Read the model definition and answer for the solid it produces. Units are mm, in the model's axes. Give positions to 0.01 mm unless a question says otherwise; leave off trailing zeros. Order: outer loops, then holes, each group sorted by start corner. A loop starts at its lowest first (then second) coordinate and runs counter-clockwise, first axis right, second up. Notation, with made-up numbers: (46, -11) - (61, -11) arc R21 ccw to (61, -1) - close; hole circle Ø3 at (80, 64.5). An arc over 180 degrees is marked (long way). Write item = value, one per line.
Autodesk Inventor part; units mm, degrees
ref_plane "YZ Plane" through (0, 0, 0) normal (1, 0, 0) x (0, 1, 0)
ref_plane "XZ Plane" through (0, 0, 0) normal (0, 1, 0) x (-1, 0, 0)
ref_plane "XY Plane" through (0, 0, 0) normal (0, 0, 1) x (1, 0, 0)
sketch "Sketch1" plane through (0, 0, 0) normal (0, 1, 0) x (-1, 0, 0)
  line L0 (0, 0) -> (100, 0)
  line L1 (100, 0) -> (100, -1220)
  line L2 (100, -1220) -> (0, -1220)
  line L3 (0, -1220) -> (0, 0)
  dimension "d0" = 100
  dimension "d1" = 1220
extrude "Extrusion1" add sketch "Sketch1" along normal blind 10
ref_plane "Work Plane1" through (-50, 0, 0) normal (1, 0, 0) x (0, 0, -1)
sketch "Sketch3" plane through (-50, 0, 0) normal (1, 0, 0) x (0, 0, -1)
  line L0 (1220, 0) -> (0, 0)
  line L1 (1220, 0) -> (1220, 10)
  line L2 (0, 10) -> (1220, 10)
  line L3 (0, 0) -> (0, 10)
  line L4 (1220, 10) -> (0, 10)
  line L5 (0, 10) -> (11.15, 10)
  circle A0 centre (11.15, 120) radius 2.5
  arc A1 (15.15, 120) -> (7.15, 120) centre (11.15, 120) ccw
  line L6 (15.15, 120) -> (15.15, 10)
  line L7 (15.15, 10) -> (7.15, 10)
  line L8 (7.15, 10) -> (7.15, 120)
  dimension "d18" = 11.15
  dimension "d21" = 5
  dimension "d22" = 8
  dimension "d24" = 8
  dimension "d31" = 110
extrude "Extrusion3" add sketch "Sketch3" along normal mid plane 10 contours L2 L8 A1 L6
sketch "Sketch4" plane through (-50, 0, 0) normal (1, 0, 0) x (0, 0, -1)
  arc A0 (15.15, 120) -> (7.15, 120) centre (11.15, 120) ccw
  circle A1 centre (11.15, 120) radius 2.5
  line L0 (7.15, 120) -> (7.15, 10)
  line L1 (15.15, 124) -> (7.15, 124)
  line L2 (7.15, 124) -> (7.15, 114)
  line L3 (7.15, 114) -> (15.15, 114)
  line L4 (15.15, 114) -> (15.15, 124)
  point P0 (0, 0)
  dimension "d27" = 10
  dimension "d30" = 4
extrude "Extrusion4" cut sketch "Sketch4" along normal mid plane 5
sketch "Sketch5" plane through (0, 10, 0) normal (0, 1, 0) x (1, 0, 0)
  line L0 (-60, 1073.331) -> (-57, 1073.331)
  line L1 (-57, 1073.331) -> (-57, 1093.331)
  line L2 (-57, 1093.331) -> (-60, 1093.331)
  line L3 (-60, 1093.331) -> (-60, 1073.331)
  line L4 (-100, 1220) -> (-100, 0)
  line L5 (0, 1220) -> (-100, 1220)
  point P0 (0, 0)
  dimension "d32" = 3
  dimension "d33" = 20
  dimension "d34" = 40
  dimension "d35" = 126.669
extrude "Extrusion5" cut sketch "Sketch5" against normal blind 10
properties part number "Base_015"
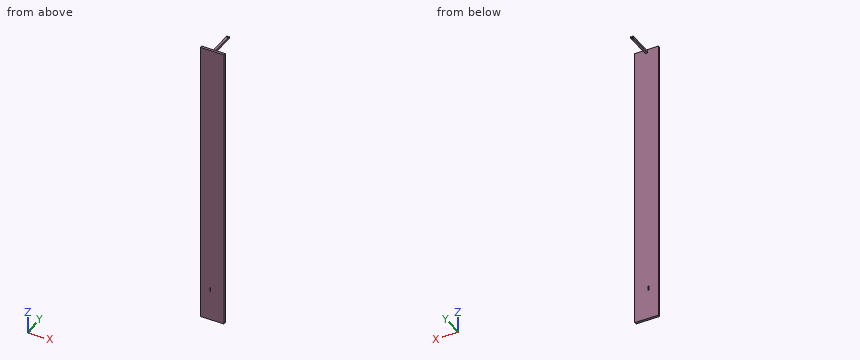
1. Flat-ended cylindrical pins translate along their axes: pin 1 (6 mm diameter, centred on y = 120, z = -11.15, fed in from +X); pin 2 (8 mm diameter, centred on y = 6, z = -1085, fed in from +X); pin 3 (5 mm diameter, centred on x = -51.5, y = 62, fed in from +Z); pin 4 (8 mm diameter, centred on x = -49, y = 92, fed in from -Z). Find the tip coordinate at first contact, or state that the pin passes through.
Recorded:
pin_1 = -45
pin_2 = 0
pin_3 = -7.15
pin_4 = -15.15
2. Section A-A (z = -753.5) is taken. Determine the outline of the cut face in (x, y).
Recorded:
outline = (-100, 0) - (0, 0) - (0, 10) - (-100, 10) - close
3. Straight lines are drawn through the part: L1, parallel to Y at x = -20, z = -928.5; L2, parallel to Y at x = -54.35, z = -11.15; L3, parallel to Z at x = -50.5, y = 80.5. For each, find the intervals that lie inside material, in ascending order. Write a range as [from, to].
Recorded:
L1 = [0, 10]
L2 = [0, 117.5], [122.5, 124]
L3 = [-15.15, -7.15]
4. Section B-B (x = -24) is taken. Determine the outline of the cut face in (y, z), and give its area (3 significant figures).
Recorded:
outline = (0, -1220) - (10, -1220) - (10, 0) - (0, 0) - close
area = 12,200 mm^2
